from build123d import *

# Parameters (mm, degrees)
SKETCH3_W           = 182.88
SKETCH3_H           = 58.42
BOSS_EXTRUDE1_DEPTH = 57.15
SKETCH4_W           = 203.2
SKETCH4_H           = 76.2
BOSS_EXTRUDE2_DEPTH = 2.54
SKETCH5_W           = 177.8
SKETCH5_H           = 53.34
CUT_EXTRUDE1_DEPTH  = 54.61
SKETCH6_R           = 2.7813
CUT_EXTRUDE2_DEPTH  = 53.34
SKETCH8_R           = 3.18135
CUT_EXTRUDE3_DEPTH  = 38.1


with BuildPart() as part:
    # Sketch3 → Boss-Extrude1 (new body)
    with BuildSketch(Plane(origin=(0, 0, 0), x_dir=(1, 0, 0), z_dir=(0, 1, 0))):
        Rectangle(SKETCH3_W, SKETCH3_H)
    extrude(amount=-BOSS_EXTRUDE1_DEPTH)

    # Sketch4 → Boss-Extrude2 (add)
    with BuildSketch(Plane(origin=(0, 0, 0), x_dir=(1, 0, 0), z_dir=(0, 1, 0))):
        Rectangle(SKETCH4_W, SKETCH4_H)
    extrude(amount=-BOSS_EXTRUDE2_DEPTH)

    # Sketch5 → Cut-Extrude1 (cut)
    with BuildSketch(Plane(origin=(0, 0, 0), x_dir=(1, 0, 0), z_dir=(0, 1, 0))):
        Rectangle(SKETCH5_W, SKETCH5_H)
    extrude(amount=-CUT_EXTRUDE1_DEPTH, mode=Mode.SUBTRACT)

    # Sketch6 → Cut-Extrude2 (cut)
    with BuildSketch(Plane(origin=(0, 0, 0), x_dir=(1, 0, 0), z_dir=(0, 1, 0))):
        with Locations((-95.25, 31.75)):
            Circle(SKETCH6_R)
        with Locations((0, 33.02)):
            Circle(SKETCH6_R)
        with Locations((95.25, 33.02)):
            Circle(SKETCH6_R)
        with Locations((95.25, -33.02)):
            Circle(SKETCH6_R)
        with Locations((0, -33.02)):
            Circle(SKETCH6_R)
        with Locations((-95.25, -31.75)):
            Circle(SKETCH6_R)
    extrude(amount=-CUT_EXTRUDE2_DEPTH, mode=Mode.SUBTRACT)

    # Sketch8 → Cut-Extrude3 (cut, symmetric)
    with BuildSketch(Plane.XY):
        with Locations((-63.5, -29.21)):
            Circle(SKETCH8_R)
    extrude(amount=CUT_EXTRUDE3_DEPTH, both=True, mode=Mode.SUBTRACT)


solid = part.part
Here's how the part is built. I have some questions about the finished solid (model axes, mm). A direction names the side the tool comes from. Round coordinates to 2 decimals unless told otherwise and drop trailing zeros. Order: outer loops, then holes, each group sorted by start corner. A loop starts at its lowest first (then second) coordinate and runs counter-clockwise, first axis right, second up. Notation, with made-up numbers: M 6.5,7 L 17.5,7 A31 cw 17.5,44 Z; hole C 65,70.25 d6. An arc over 180 degrees is marked long. Return JSON: item names as keys, results as strings. Group by question number.
1. If we mould it in two halves opening along Z, with no side actions, what happens to faces 1 (the face through (-1, -29, -29.21)), 2 (the face through (97.819, -1.252, -31.955)), 3 (the face through (0, 0, 28))? For each: pulls with the +Z half, pulls with the -Z half, needs draft (parallel to the pull), parting line crosses it, or undercut.
2. On a 3-axis mill with a long thin cutter (end or side, diameter ignored), from which of +Z, -Z, +X, -X, +Y, -Y can I reach the whole of each face in a straight line? I mean faces 4 (the face through (-91.44, -29, 0)), 5 (the face through (-1, -29, 29.21)), 6 (the face through (-1, -27, 26.67)), 7 (the face through (91.44, -29, 0)). Say none if no direction works.
3. If we section it at B-B on z = -9.5: List the corners of the cut face in (x, y) for me, then the cut area to 3 significant figures.
4. If we section it at D-D on x = 0: List the corners of the cut face in (y, z) for me, then the cut area to 3 significant figures.
5. I'm going to push flat-ended pins straight in: pin 1 Ø4 at (x, y) = (-63.5, -29.21) entering from -Z; pin 2 Ø9 at (x, z) = (95.25, -33.02) entering from -Y; pin 3 Ø4 at (y, z) = (-26.5, -18.5) entering from -X; pin 4 Ø5 at (x, y) = (60, -48) entering from -Z. Where does each tip first touch, or does it pass through?
6. If we section it at C-C on y = -46: List the corners of the cut face in (x, z) for me, then the cut area to 3 significant figures.
7. If we section it at A-A on x = 95.25: List the corners of the cut face in (y, z) for me, then the cut area to 3 significant figures.
8. Please list where these lines run through material, in increasing order: probe 1 along Z at (x, y) = (9.5, -18); probe 2 along Z at (x, y) = (61.5, -2.5); probe 3 along X at (y, z) = (-52, -4).
Reply:
{
 "1": {"face 1": "pulls with the -Z half", "face 2": "undercut", "face 3": "needs draft"},
 "2": {"face 4": "+Z, -Z, -X, -Y", "face 5": "+Z, +X, -X, -Y", "face 6": "+Y", "face 7": "+Z, -Z, +X, -Y"},
 "3": {"outline": "M -101.6,-2.54 L -91.44,-2.54 L -91.44,-57.15 L 91.44,-57.15 L 91.44,-2.54 L 101.6,-2.54 L 101.6,0 L 88.9,0 L 88.9,-54.61 L -88.9,-54.61 L -88.9,0 L -101.6,0 Z", "area": "794 mm^2"},
 "4": {"outline": "M -57.15,-29.21 L -2.54,-29.21 L -2.54,-30.24 L 0,-30.24 L 0,-26.67 L -54.61,-26.67 L -54.61,26.67 L 0,26.67 L 0,30.24 L -2.54,30.24 L -2.54,29.21 L -57.15,29.21 Z; M -2.54,-38.1 L 0,-38.1 L 0,-35.8 L -2.54,-35.8 Z; M -2.54,35.8 L 0,35.8 L 0,38.1 L -2.54,38.1 Z", "area": "443 mm^2"},
 "5": {"pin 1": "through", "pin 2": "y = -2.54", "pin 3": "x = -91.44", "pin 4": "z = -29.21"},
 "6": {"outline": "M -91.44,-29.21 L 91.44,-29.21 L 91.44,29.21 L -91.44,29.21 Z; hole M -88.9,-26.67 L 88.9,-26.67 L 88.9,26.67 L -88.9,26.67 Z", "area": "1,200 mm^2"},
 "7": {"outline": "M -2.54,-38.1 L 0,-38.1 L 0,-35.8 L -2.54,-35.8 Z; M -2.54,-30.24 L 0,-30.24 L 0,30.24 L -2.54,30.24 Z; M -2.54,35.8 L 0,35.8 L 0,38.1 L -2.54,38.1 Z", "area": "165 mm^2"},
 "8": {"probe 1": "-29.21 to -26.67, 26.67 to 29.21", "probe 2": "-38.1 to -26.67, 26.67 to 38.1", "probe 3": "-91.44 to -88.9, 88.9 to 91.44"}
}
